```python
from build123d import *

# Parameters (mm, degrees)
F0_W     = 152.4
F0_H     = 152.4
F1_DEPTH = 152.4
F2_W     = 114.3
F2_H     = 114.3
F3_DEPTH = 152.4
F4_W     = 101.6
F4_H     = 50.8
F5_DEPTH = 127
F6_W     = 50.8
F6_H     = 101.6
F7_DEPTH = 127


with BuildPart() as f1:
    # F0 (on Front) → F1 (new body)
    with BuildSketch(Plane.XZ):
        with Locations((76.2, 76.2)):
            Rectangle(F0_W, F0_H)
    extrude(amount=F1_DEPTH)

    # F2 (on face) → F3 (cut)
    with BuildSketch(Plane.XZ.offset(152.4)):
        with Locations((95.25, 95.25)):
            Rectangle(F2_W, F2_H)
    extrude(amount=-F3_DEPTH, mode=Mode.SUBTRACT)

    # F4 (on face) → F5 (cut)
    with BuildSketch(Plane.XY.offset(38.1)):
        with Locations((152.4, -76.2)):
            Rectangle(F4_W, F4_H)
    extrude(amount=-F5_DEPTH, mode=Mode.SUBTRACT)

    # F6 (on face) → F7 (cut)
    with BuildSketch(Plane.YZ.offset(38.1)):
        with Locations((-76.2, 152.4)):
            Rectangle(F6_W, F6_H)
    extrude(amount=-F7_DEPTH, mode=Mode.SUBTRACT)


solid = f1.part
```
Work out the finished part from the listing and answer in its coordinate system (mm). A direction names the side the tool comes from. Give positions to 0.01 mm unless a question says otherwise; leave off trailing zeros. Loops run counter-clockwise (first coordinate to the right, second up) from the corner with the lowest first, then second, coordinate; pieces in that order, holes last. Notation, with made-up numbers: (11, -22.75) - (61, -22.75) arc R34 ccw to (61, 13.25) - close; hole circle Ø9 at (-2, 72.25). An arc over 180 degrees is marked (long way). One line per question, with ' | ' between items.
(1) The mould has two halves that part along Y. Classify faces 1 (the face through (19, -77, 101.6)), 2 (the face through (24, -152.4, 43)), 3 (the face through (24, 0, 43)), 4 (the face through (101.6, -77, 19)): +Y half, -Y half, draft (parallel to the pull), parting line (faces both ways), or undercut.
Recorded:
face 1: undercut | face 2: -Y half | face 3: +Y half | face 4: undercut
(2) The part is cut by section B-B (x = 108.5). Write down the section's boundary in (y, z).
Recorded:
outline: (-152.4, 0) - (-101.6, 0) - (-101.6, 38.1) - (-152.4, 38.1) - close; (-50.8, 0) - (0, 0) - (0, 38.1) - (-50.8, 38.1) - close
(3) The part is cut by section C-C (z = 33). Write down the section's boundary in (x, y).
Recorded:
outline: (0, -152.4) - (152.4, -152.4) - (152.4, -101.6) - (101.6, -101.6) - (101.6, -50.8) - (152.4, -50.8) - (152.4, 0) - (0, 0) - close
(4) Each of these flat-tipped pins is pushed along its axis until it touches: pin 1 Ø10 at (x, y) = (45.5, -121) entering from +Z; pin 2 Ø19 at (y, z) = (-79.5, 14.5) entering from +X. Where does it stop, or does it pass through?
Recorded:
pin 1: stops at z = 38.1 | pin 2: stops at x = 101.6
(5) Straight lines are drawn through the part: probe 1 along Y at (x, z) = (14.5, 143); probe 2 along Z at (x, y) = (110, -27.5). For each, find the intervals that lie inside material, in ascending order.
Recorded:
probe 1: y = -152.4 to -101.6, -50.8 to 0 | probe 2: z = 0 to 38.1
(6) The part is cut by section D-D (y = -70.5). Write down the section's boundary in (x, z), then the cut area to 3 significant figures.
Recorded:
outline: (0, 0) - (101.6, 0) - (101.6, 38.1) - (38.1, 38.1) - (38.1, 101.6) - (0, 101.6) - close | area: 6,290 mm²
(7) A tool of negligible diameter and unlimited length cuts with its end or side. For faces 5 (the face through (127, -50.8, 19)), 6 (the face through (38.1, -77, 94)), 7 (the face through (19, -101.6, 127)), from which of +Z, -Z, +X, -X, +Y, -Y can it reach the whole face along a straight path? Write none if from no direction.
Recorded:
face 5: +Z, -Z, +X | face 6: +Z, +X, +Y, -Y | face 7: +Z, +X, -X
(8) The part is cut by section A-A (z = 111). Write down the section's boundary in (x, y).
Recorded:
outline: (0, -152.4) - (38.1, -152.4) - (38.1, -101.6) - (0, -101.6) - close; (0, -50.8) - (38.1, -50.8) - (38.1, 0) - (0, 0) - close
